The listing builds one solid part. Answer for the finished solid, in the listing's coordinates (mm). A direction names the side the tool comes from. Round coordinates to 2 decimals unless told otherwise and drop trailing zeros. Loops run counter-clockwise (first coordinate to the right, second up) from the corner with the lowest first, then second, coordinate; pieces in that order, holes last. Notation, with made-up numbers: M 33.25,-28.75 L 45.25,-28.75 A9 ccw 45.25,-11.75 Z; hole C -12,80 d11. An arc over 180 degrees is marked long. Put each result on its own line as item: value. Start each with the question number.
(1) A flat-ended cylindrical pin translates along its axis: P1, Ø13, axis at x = 261, z = 22, coming from the +Y side. Find the tip coordinate at first contact, or state that the pin passes through.
(2) Which of the six approach directions +Z, -Z, +X, -X, +Y, -Y give full straight-line access (tool end or side, diameter ignored) to faces 5 (the face through (321, 22, 44)), 6 (the face through (318, 19, 50))?
(3) Section C-C, the plane y = 30.5 is taken. Determine the outline of the cut face in (x, z), then the cut area to 3 significant figures.
(4) Determine the mould class of faces 1 (the face through (633, 13, 45)), 2 (the face through (631.584, -3.042, 24.703)), 3 (the face through (319, -6, 25)), 4 (the face through (10, -3, 10)) for opening direction X: released by +X, released by -X, zero draft, split by the parting line, or undercut.
(5) Straight lines are drawn through the part: line 1 (Z direction, x = 25, y = -2); line 2 (Y direction, x = 75, z = 25.5); line 3 (Z direction, x = 74, y = 2.5). For each, find the intervals that lie inside material, in ascending order.
(6) Section B-B, the plane x = 534.5 is taken. Determine the outline of the cut face in (y, z).
(7) Section A-A, the plane z = 6.5 is taken. Determine the outline of the cut face in (x, y).
```python
from build123d import *

# Parameters (mm, degrees)
F0_W     = 648
F0_H     = 50
F1_DEPTH = 6
F2_W     = 648
F2_H     = 6
F3_DEPTH = 44
F4_R     = 9
F5_DEPTH = 50.001


with BuildPart() as f1:
    # F0 (on Front) → F1 (new body)
    with BuildSketch(Plane.XZ):
        with Locations((324, 25)):
            Rectangle(F0_W, F0_H)
    extrude(amount=F1_DEPTH)

    # F2 (on face) → F3 (join)
    with BuildSketch(Plane(origin=(0, 0, 0), x_dir=(-1, 0, 0), z_dir=(0, 1, 0))):
        with Locations((-324, 47)):
            Rectangle(F2_W, F2_H)
    extrude(amount=F3_DEPTH)

    # F4 (on face) → F5 (cut, through all)
    with BuildSketch(Plane.XZ.offset(6)):
        Polygon((20, 0), (0, 20), (0, 0), align=None)
        Polygon((628, 50), (648, 30), (648, 50), align=None)
        with Locations((25, 22)):
            Circle(F4_R)
        with Locations((623, 22)):
            Circle(F4_R)
    extrude(amount=-F5_DEPTH, mode=Mode.SUBTRACT)


solid = f1.part
```
Recorded:
1. P1: stops at y = 0
2. face 5: -Z, +X, -X, +Y
2. face 6: +Z, +X, -X, +Y, -Y
3. outline: M 0,44 L 634,44 L 628,50 L 0,50 Z
3. area: 3,790 mm²
4. face 1: released by +X
4. face 2: undercut
4. face 3: zero draft
4. face 4: released by -X
5. line 1: z = 0 to 13, 31 to 50
5. line 2: y = -6 to 0
5. line 3: z = 44 to 50
6. outline: M -6,0 L 0,0 L 0,44 L 44,44 L 44,50 L -6,50 Z
7. outline: M 13.5,-6 L 648,-6 L 648,0 L 13.5,0 Z
